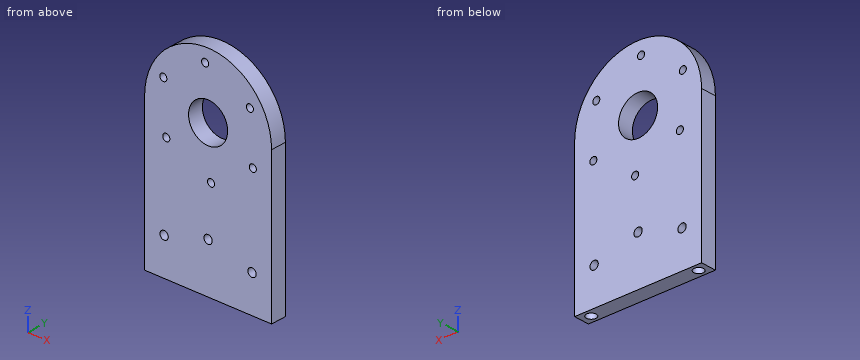
from build123d import *

# Parameters (mm, degrees)
PARED_A_MOTOR_J5_START           = 50.525
CROQUIS1_W                       = 52
CROQUIS1_H                       = 60.6
PARED_A_MOTOR_J5_DEPTH           = 6.35
PARED_A_MOTOR_J5_REDONDEO_START  = 50.525
CROQUIS2_R                       = 26
PARED_A_MOTOR_J5_REDONDEO_DEPTH  = 6.35
BARRENOS_M5_START                = 50.525
CROQUIS3_R                       = 1.45
CROQUIS3_R_2                     = 8
BARRENOS_M5_DEPTH                = 6.35
ROSCA_M3_ESCUADRAS_START         = 50.525
CROQUIS4_R                       = 1.25
ROSCA_M3_ESCUADRAS_DEPTH         = 6.35
PASADORES_D4_START               = 275.95
CROQUIS5_R                       = 2
PASADORES_D4_DEPTH               = 8
ROSCA_M3_BASES_CINCHO_START      = 50.525
CROQUIS6_R                       = 1.25
ROSCA_M3_BASES_CINCHO_DEPTH      = 6.35
PASO_M3_ESCUADRAS_TUERCA_START   = 50.525
CROQUIS7_R                       = 1.7
PASO_M3_ESCUADRAS_TUERCA_DEPTH   = 6.35
PASO_M3_BASE_CINCHO_TUERCA_START = 50.525
CROQUIS8_R                       = 1.7
PASO_M3_BASE_CINCHO_TUERCA_DEPTH = 6.35


with BuildPart() as part:
    # Croquis1 → Pared_A_motor_J5 (new body)
    with BuildSketch(Plane(origin=(0, 0, 0), x_dir=(1, 0, 0), z_dir=(0, 1, 0)).offset(PARED_A_MOTOR_J5_START)):
        with Locations((152.4, -306.25)):
            Rectangle(CROQUIS1_W, CROQUIS1_H)
    extrude(amount=PARED_A_MOTOR_J5_DEPTH)

    # Croquis2 → Pared_A_motor_J5_redondeo (add)
    with BuildSketch(Plane(origin=(0, 0, 0), x_dir=(1, 0, 0), z_dir=(0, 1, 0)).offset(PARED_A_MOTOR_J5_REDONDEO_START)):
        with Locations((152.4, -336.55)):
            Circle(CROQUIS2_R)
    extrude(amount=PARED_A_MOTOR_J5_REDONDEO_DEPTH)

    # Croquis3 → Barrenos_M5 (cut)
    with BuildSketch(Plane(origin=(0, 0, 0), x_dir=(1, 0, 0), z_dir=(0, 1, 0)).offset(BARRENOS_M5_START)):
        with Locations(Location((169.514381197, -347.834855172, 0), (0, 0, 270))):
            Circle(CROQUIS3_R)
        with Locations(Location((151.184219342, -357.013916472, 0), (0, 0, 270))):
            Circle(CROQUIS3_R)
        with Locations(Location((134.069838145, -345.729061301, 0), (0, 0, 270))):
            Circle(CROQUIS3_R)
        with Locations(Location((135.285618803, -325.265144828, 0), (0, 0, 270))):
            Circle(CROQUIS3_R)
        with Locations(Location((153.615780658, -316.086083528, 0), (0, 0, 270))):
            Circle(CROQUIS3_R)
        with Locations(Location((170.730161855, -327.370938699, 0), (0, 0, 270))):
            Circle(CROQUIS3_R)
        with Locations(Location((152.4, -336.55, 0), (0, 0, 270))):
            Circle(CROQUIS3_R_2)
    extrude(amount=BARRENOS_M5_DEPTH, mode=Mode.SUBTRACT)

    # Croquis4 → Rosca_M3_escuadras (cut)
    with BuildSketch(Plane(origin=(0, 0, 0), x_dir=(1, 0, 0), z_dir=(0, 1, 0)).offset(ROSCA_M3_ESCUADRAS_START)):
        with Locations(Location((134.4, -290.95, 0), (0, 0, 270))):
            Circle(CROQUIS4_R)
        with Locations(Location((170.4, -290.95, 0), (0, 0, 270))):
            Circle(CROQUIS4_R)
    extrude(amount=ROSCA_M3_ESCUADRAS_DEPTH, mode=Mode.SUBTRACT)

    # Croquis5 → Pasadores_D4 (cut)
    with BuildSketch(Plane.XY.offset(PASADORES_D4_START)):
        with Locations((130.4, 53.7)):
            Circle(CROQUIS5_R)
        with Locations((174.4, 53.7)):
            Circle(CROQUIS5_R)
    extrude(amount=PASADORES_D4_DEPTH, mode=Mode.SUBTRACT)

    # Croquis6 → Rosca_M3_bases_cincho (cut)
    with BuildSketch(Plane(origin=(0, 0, 0), x_dir=(1, 0, 0), z_dir=(0, 1, 0)).offset(ROSCA_M3_BASES_CINCHO_START)):
        with Locations(Location((152.4, -296, 0), (0, 0, 270))):
            Circle(CROQUIS6_R)
    extrude(amount=ROSCA_M3_BASES_CINCHO_DEPTH, mode=Mode.SUBTRACT)

    # Croquis7 → Paso_M3_escuadras_tuerca (cut)
    with BuildSketch(Plane(origin=(0, 0, 0), x_dir=(1, 0, 0), z_dir=(0, 1, 0)).offset(PASO_M3_ESCUADRAS_TUERCA_START)):
        with Locations(Location((134.4, -290.95, 0), (0, 0, 270))):
            Circle(CROQUIS7_R)
        with Locations(Location((170.4, -290.95, 0), (0, 0, 270))):
            Circle(CROQUIS7_R)
    extrude(amount=PASO_M3_ESCUADRAS_TUERCA_DEPTH, mode=Mode.SUBTRACT)

    # Croquis8 → Paso_M3_base_cincho_tuerca (cut)
    with BuildSketch(Plane(origin=(0, 0, 0), x_dir=(1, 0, 0), z_dir=(0, 1, 0)).offset(PASO_M3_BASE_CINCHO_TUERCA_START)):
        with Locations(Location((152.4, -296, 0), (0, 0, 270))):
            Circle(CROQUIS8_R)
    extrude(amount=PASO_M3_BASE_CINCHO_TUERCA_DEPTH, mode=Mode.SUBTRACT)


solid = part.part
Design review of the part built by this model. Coordinates are the model's own, in mm. Round coordinates to 2 decimals unless told otherwise and drop trailing zeros. Write each loop counter-clockwise with the first axis right and the second up, starting at its lowest first coordinate (ties: lowest second). Pieces come first, ordered by that corner, then holes. Notation, with made-up numbers: M 48,40 L 72,40 A26 cw 72,75 Z; hole C -28.5,45.5 d5. An arc over 180 degrees is marked long. One line per item, written item: value. Start each with the question number.
1. Take a section at B-B on y = 53.7. State how many separate pieces and enclosed holes the cut face has, then the cut area to 3 significant figures.
2. Clearance check with flat-ended pins moving along their axes: P1, Ø1, axis at x = 140, y = 52.5, coming from the +Z side; P2, Ø1.2, axis at x = 131, y = 53.5, coming from the -Z side; P3, Ø1, axis at x = 144.5, y = 53.5, coming from the +Z side. State where each tip first meets the part, or that it passes through.
3. Take a section at C-C on x = 157.5. State the section outline as (y, z) points (3 decimals).
4. Take a section at A-A on z = 290.95. State the section outline as (x, y) points (3 decimals).
5. Take a section at D-D on x = 130.4. State the section outline as (y, z) points (3 decimals), then the cut area to 3 significant figures.
6. To check wall thickness, follow probe 1 along Z at (x, y) = (134.4, 54.75); probe 2 along X at (y, z) = (56.75, 291); probe 3 along X at (y, z) = (52.75, 281.5). State the ranges of each line that lie inside material, in increasing order. Write a range as from..to.
Computed:
1. separate pieces: 1
1. enclosed holes: 10
1. area: 3,880 mm²
2. P1: stops at z = 359.67
2. P2: stops at z = 283.95
2. P3: stops at z = 361.47
3. outline: M 50.525,275.95 L 56.875,275.95 L 56.875,330.386 L 50.525,330.386 Z; M 50.525,342.714 L 56.875,342.714 L 56.875,362.045 L 50.525,362.045 Z
4. outline: M 126.4,50.525 L 132.7,50.525 L 132.7,56.875 L 126.4,56.875 Z; M 136.1,50.525 L 168.7,50.525 L 168.7,56.875 L 136.1,56.875 Z; M 172.1,50.525 L 178.4,50.525 L 178.4,56.875 L 172.1,56.875 Z
5. outline: M 50.525,275.95 L 51.7,275.95 L 51.7,283.95 L 55.7,283.95 L 55.7,275.95 L 56.875,275.95 L 56.875,350.406 L 50.525,350.406 Z
5. area: 441 mm²
6. probe 1: z = 275.95..289.25, 292.65..324.12, 326.41..344.32, 347.14..355.31
6. probe 2: x = 126.4..132.7, 136.1..168.7, 172.1..178.4
6. probe 3: x = 126.4..128.64, 132.16..172.64, 176.16..178.4
